The drawing under review shows one solid part. Ordinate dimensions are in mm from its lowest x, y, z. A direction names the side the tool comes from. Coordinates: 2 decimals unless noted, no trailing zeros. Order: outer loops, then holes, each group sorted by start corner. A loop starts at its lowest first (then second) coordinate and runs counter-clockwise, first axis right, second up. Notation, with made-up numbers: (-14.5, 83.25) - (6.5, 83.25) arc R17 ccw to (6.5, 102.25) - close; hole circle Ø8 at (72.5, -8). An arc over 180 degrees is marked (long way). Answer in a Markdown table with one row per item.
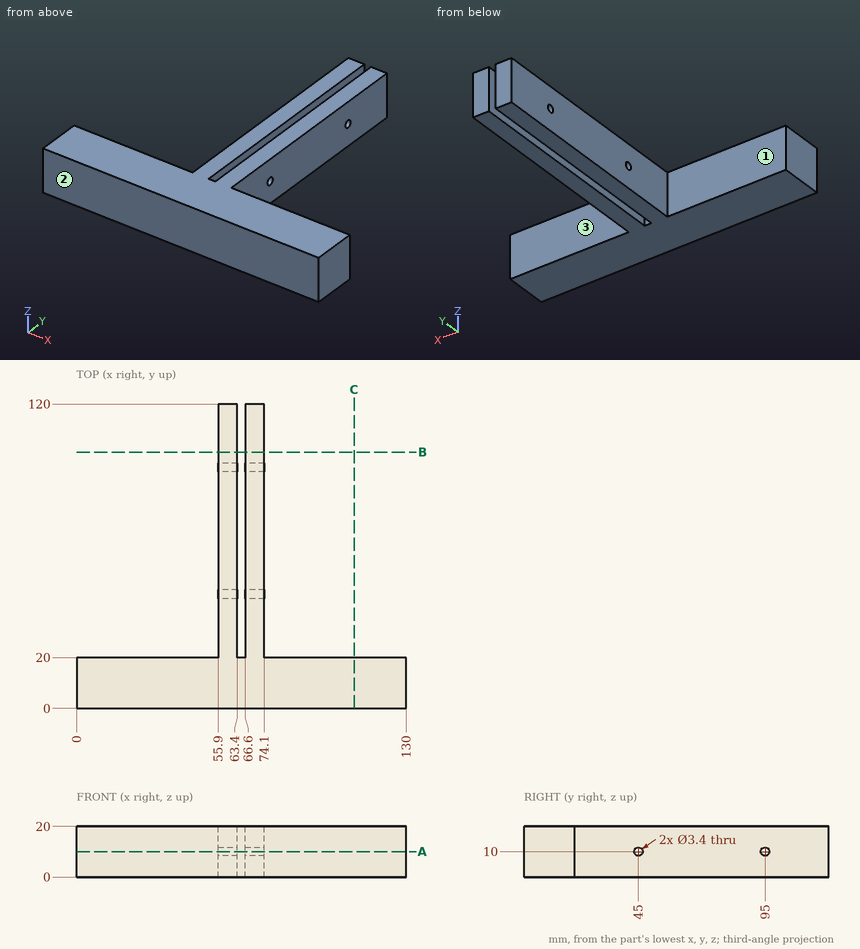
Item 1: We need section C-C, the plane x = 109.5. Write out the cut boundary in (y, z), then the cut area to 3 significant figures.
Check values:
| item | result |
|---|---|
| outline | (0, 0) - (20, 0) - (20, 20) - (0, 20) - close |
| area | 400 mm^2 |
Item 2: Tool access review of the marked faces 1, 2 and 3: name each direction out of +Z, -Z, +X, -X, +Y, -Y from which nothing blocks a thin tool from reaching the whole face with its end or side.
Check values:
| item | result |
|---|---|
| face 1 | +Z, -Z, -X, +Y |
| face 2 | +Z, -Z, +X, -X, -Y |
| face 3 | +Z, -Z, +X, +Y |
Item 3: We need section A-A, the plane z = 10. Write out the cut boundary in (x, y).
Check values:
| item | result |
|---|---|
| outline | (0, 0) - (130, 0) - (130, 20) - (74.1, 20) - (74.1, 43.3) - (66.6, 43.3) - (66.6, 20) - (63.4, 20) - (63.4, 43.3) - (55.9, 43.3) - (55.9, 20) - (0, 20) - close; (55.9, 46.7) - (63.4, 46.7) - (63.4, 93.3) - (55.9, 93.3) - close; (55.9, 96.7) - (63.4, 96.7) - (63.4, 120) - (55.9, 120) - close; (66.6, 46.7) - (74.1, 46.7) - (74.1, 93.3) - (66.6, 93.3) - close; (66.6, 96.7) - (74.1, 96.7) - (74.1, 120) - (66.6, 120) - close |
Item 4: Clearance check with flat-ended pins moving along their axes: pin 1 Ø10 at (y, z) = (54.5, 14) entering from -X; pin 2 Ø1 at (x, z) = (23.5, 15.5) entering from -Y; pin 3 Ø1 at (y, z) = (60.5, 15.5) entering from +X; pin 4 Ø2 at (y, z) = (95, 10) entering from +X. State where each tip first meets the part, or that it passes through.
Check values:
| item | result |
|---|---|
| pin 1 | x = 55.9 |
| pin 2 | y = 0 |
| pin 3 | x = 74.1 |
| pin 4 | through |
Item 5: To check wall thickness, follow line 1 (Y direction, x = 72, z = 10); line 2 (Z direction, x = 68.75, y = 95); line 3 (X direction, y = 90, z = 17). State the ranges of each line that lie inside material, in increasing order. Write a range as from..to.
Check values:
| item | result |
|---|---|
| line 1 | 0..43.3, 46.7..93.3, 96.7..120 |
| line 2 | 0..8.3, 11.7..20 |
| line 3 | 55.9..63.4, 66.6..74.1 |
Item 6: We need section B-B, the plane y = 101. Write out the cut boundary in (x, z).
Check values:
| item | result |
|---|---|
| outline | (55.9, 0) - (63.4, 0) - (63.4, 20) - (55.9, 20) - close; (66.6, 0) - (74.1, 0) - (74.1, 20) - (66.6, 20) - close |
